```python
from build123d import *

# Parameters (mm, degrees)
SKETCH3_W                       = 111.348371095
SKETCH3_H                       = 23.1
BOSS_EXTRUDE1_DEPTH             = 5
SKETCH3_4_W                     = 34.9
SKETCH3_4_H                     = 23.1
BOSS_EXTRUDE2_DEPTH             = 2.5
CUT_EXTRUDE1_DEPTH              = 30.8
CUT_EXTRUDE1_DEPTH_BACK         = 67.894637304
SKETCH4_4_R                     = 12.7
BOSS_EXTRUDE3_START             = -1
SKETCH4_R                       = 12.7
SKETCH4_R_2                     = 4
SKETCH4_R_3                     = 1.6
BOSS_EXTRUDE3_DEPTH             = 2
BOSS_EXTRUDE4_DEPTH             = 2
BOSS_EXTRUDE4_DEPTH_BACK        = 13
BOSS_EXTRUDE4_START             = -3
SKETCH4_3_R                     = 14.8
SKETCH4_3_R_2                   = 12.7
BOSS_EXTRUDE6_REACH             = 105.413
SKETCH6_R                       = 1.7
BOSS_EXTRUDE6_DIRECTION_2_REACH = 105.413
CUT_EXTRUDE5_START              = -9.55
SKETCH6_9_R                     = 1.7
CUT_EXTRUDE5_DEPTH              = 19.1
FILLET1_R                       = 3
SKETCH12_W                      = 31.185762671
SKETCH12_H                      = 41.424107397
CUT_EXTRUDE9_DEPTH              = 2.9
FILLET2_R                       = 1
CUT_EXTRUDE10_DEPTH             = 108.072038083
FILLET3_R                       = 2
SKETCH14_W                      = 6
SKETCH14_H                      = 8
SKETCH14_R                      = 1.75
BOSS_EXTRUDE8_DEPTH             = 5
FILLET4_R                       = 10


with BuildPart() as part:
    # Sketch3 → Boss-Extrude1 (new body)
    with BuildSketch(Plane(origin=(0, 0, 0), x_dir=(1, 0, 0), z_dir=(0, 1, 0))):
        with Locations((-43.674185548, 0)):
            Rectangle(SKETCH3_W, SKETCH3_H)
    extrude(amount=-BOSS_EXTRUDE1_DEPTH)

    # Sketch3<4> → Boss-Extrude2 (add)
    with BuildSketch(Plane(origin=(0, 0, 0), x_dir=(1, 0, 0), z_dir=(0, 1, 0))):
        with Locations((-5.45, 0)):
            Rectangle(SKETCH3_4_W, SKETCH3_4_H)
        Polygon((-20.2, 9.55), (9.3, 9.55), (10, 9.55), (10, -9.55), (9.3, -9.55), (-20.2, -9.55), (-20.9, -9.55), (-20.9, 9.55), align=None, mode=Mode.SUBTRACT)
    extrude(amount=BOSS_EXTRUDE2_DEPTH)

    # Sketch4<4> → Cut-Extrude1 (cut, two sides: drawn at the far end of the back side and taken through both)
    with BuildSketch(Plane(origin=(-53.7, 0, 0), x_dir=(0, 0, -1), z_dir=(1, 0, 0)).offset(-CUT_EXTRUDE1_DEPTH_BACK)):
        with Locations((0, 9.8)):
            Circle(SKETCH4_4_R)
    extrude(amount=CUT_EXTRUDE1_DEPTH + CUT_EXTRUDE1_DEPTH_BACK, mode=Mode.SUBTRACT)

    # Sketch4 → Boss-Extrude3 (add)
    with BuildSketch(Plane(origin=(-53.7, 0, 0), x_dir=(0, 0, -1), z_dir=(1, 0, 0)).offset(BOSS_EXTRUDE3_START)):
        with Locations((0, 9.8)):
            Circle(SKETCH4_R)
        with Locations((0, 9.8)):
            Circle(SKETCH4_R_2, mode=Mode.SUBTRACT)
        with Locations((0, 18.3)):
            Circle(SKETCH4_R_3, mode=Mode.SUBTRACT)
        with Locations((0, 1.3)):
            Circle(SKETCH4_R_3, mode=Mode.SUBTRACT)
    extrude(amount=-BOSS_EXTRUDE3_DEPTH)

    # Sketch4<3> → Boss-Extrude4 (add, two sides: drawn at the far end of the back side and taken through both)
    with BuildSketch(Plane(origin=(-53.7, 0, 0), x_dir=(0, 0, -1), z_dir=(1, 0, 0)).offset(BOSS_EXTRUDE4_START - BOSS_EXTRUDE4_DEPTH_BACK)):
        with Locations((0, 9.8)):
            Circle(SKETCH4_3_R)
        with Locations((0, 9.8)):
            Circle(SKETCH4_3_R_2, mode=Mode.SUBTRACT)
    extrude(amount=BOSS_EXTRUDE4_DEPTH + BOSS_EXTRUDE4_DEPTH_BACK)

    # Boss-Extrude6: up to this face of the body (flat: up to its plane)
    boss_extrude6_end = Plane(part.part.faces().sort_by_distance((-38.495455163, -1.99193845, 11.55))[0])
    # Sketch6 → Boss-Extrude6 (add, up to the picked face)
    with BuildSketch(Plane.XY, mode=Mode.PRIVATE) as boss_extrude6_sk1:
        with BuildLine():
            Line((-22.9, 2.5), (-22.9, 3))
            ThreePointArc((-22.9, 3), (-21.435533906, 6.535533906), (-17.9, 8))
            Line((-17.9, 8), (-8.9, 8))
            Line((-8.9, 8), (0, 8))
            Line((0, 8), (0, 29))
            ThreePointArc((0, 29), (0.292893219, 29.707106781), (1, 30))
            Line((1, 30), (11, 30))
            ThreePointArc((11, 30), (11.707106781, 29.707106781), (12, 29))
            Line((12, 29), (12, 2.5))
            Line((12, 2.5), (12, 0))
            Line((12, 0), (10, 0))
            Line((10, 0), (10, 2.5))
            Line((10, 2.5), (-22.9, 2.5))
        make_face()
        with Locations(Location((-15.9, 4.5, 0), (0, 0, 180))):
            Circle(SKETCH6_R, mode=Mode.SUBTRACT)
        with Locations(Location((4.6, 25, 0), (0, 0, 180))):
            Circle(SKETCH6_R, mode=Mode.SUBTRACT)
    boss_extrude6_tool1 = split(extrude(boss_extrude6_sk1.sketch, amount=BOSS_EXTRUDE6_REACH, mode=Mode.PRIVATE), bisect_by=boss_extrude6_end, keep=Keep.BOTH, mode=Mode.PRIVATE)
    add(boss_extrude6_tool1.solids().sort_by(Axis((1.853009, 13.07203, 0), (0, 0, 1)))[0])

    # Boss-Extrude6 direction 2: up to this face of the body (flat: up to its plane)
    boss_extrude6_direction_2_end = Plane(part.part.faces().sort_by_distance((-38.495455163, -1.99193845, -11.55))[0])
    # Sketch6 → Boss-Extrude6 direction 2 (add, up to the picked face)
    with BuildSketch(Plane.XY, mode=Mode.PRIVATE) as boss_extrude6_direction_2_sk1:
        with BuildLine():
            Line((-22.9, 2.5), (-22.9, 3))
            ThreePointArc((-22.9, 3), (-21.435533906, 6.535533906), (-17.9, 8))
            Line((-17.9, 8), (-8.9, 8))
            Line((-8.9, 8), (0, 8))
            Line((0, 8), (0, 29))
            ThreePointArc((0, 29), (0.292893219, 29.707106781), (1, 30))
            Line((1, 30), (11, 30))
            ThreePointArc((11, 30), (11.707106781, 29.707106781), (12, 29))
            Line((12, 29), (12, 2.5))
            Line((12, 2.5), (12, 0))
            Line((12, 0), (10, 0))
            Line((10, 0), (10, 2.5))
            Line((10, 2.5), (-22.9, 2.5))
        make_face()
        with Locations(Location((-15.9, 4.5, 0), (0, 0, 180))):
            Circle(SKETCH6_R, mode=Mode.SUBTRACT)
        with Locations(Location((4.6, 25, 0), (0, 0, 180))):
            Circle(SKETCH6_R, mode=Mode.SUBTRACT)
    boss_extrude6_direction_2_tool1 = split(extrude(boss_extrude6_direction_2_sk1.sketch, amount=-BOSS_EXTRUDE6_DIRECTION_2_REACH, mode=Mode.PRIVATE), bisect_by=boss_extrude6_direction_2_end, keep=Keep.BOTH, mode=Mode.PRIVATE)
    add(boss_extrude6_direction_2_tool1.solids().sort_by(Axis((1.853009, 13.07203, 0), (0, 0, -1)))[0])

    # Sketch6<9> → Cut-Extrude5 (cut)
    with BuildSketch(Plane.XY.offset(CUT_EXTRUDE5_START)):
        with BuildLine():
            Line((-22.9, 2.5), (-22.9, 3))
            ThreePointArc((-22.9, 3), (-21.435533906, 6.535533906), (-17.9, 8))
            Line((-17.9, 8), (-8.9, 8))
            Line((-8.9, 8), (0, 8))
            Line((0, 8), (0, 29))
            ThreePointArc((0, 29), (0.292893219, 29.707106781), (1, 30))
            Line((1, 30), (11, 30))
            ThreePointArc((11, 30), (11.707106781, 29.707106781), (12, 29))
            Line((12, 29), (12, 2.5))
            Line((12, 2.5), (12, 0))
            Line((12, 0), (10, 0))
            Line((10, 0), (10, 2.5))
            Line((10, 2.5), (-22.9, 2.5))
        make_face()
        with Locations(Location((-15.9, 4.5, 0), (0, 0, 180))):
            Circle(SKETCH6_9_R, mode=Mode.SUBTRACT)
        with Locations(Location((4.6, 25, 0), (0, 0, 180))):
            Circle(SKETCH6_9_R, mode=Mode.SUBTRACT)
    extrude(amount=CUT_EXTRUDE5_DEPTH, mode=Mode.SUBTRACT)

    # Fillet1
    fillet1_edges = [part.edges().sort_by_distance(p)[0] for p in [
        (0, 8, -10.55),
        (0, 8, 10.55),
    ]]
    fillet(fillet1_edges, radius=FILLET1_R)

    # Sketch12 → Cut-Extrude9 (cut)
    with BuildSketch(Plane(origin=(12, 0, 0), x_dir=(0, 0, -1), z_dir=(1, 0, 0))):
        with Locations((1.113943618, 12.240146633)):
            Rectangle(SKETCH12_W, SKETCH12_H)
    extrude(amount=-CUT_EXTRUDE9_DEPTH, mode=Mode.SUBTRACT)

    # Fillet2
    fillet2_edges = [part.edges().sort_by_distance(p)[0] for p in [
        (9.1, 30, 10.55),
        (9.1, 30, -10.55),
    ]]
    fillet(fillet2_edges, radius=FILLET2_R)

    # Sketch13 → Cut-Extrude10 (cut, through all)
    with BuildSketch(Plane(origin=(0, 0, -11.55), x_dir=(-1, 0, 0), z_dir=(0, 0, -1))):
        Polygon((-4.55, 30), (0, 25), (0, 30), align=None)
    extrude(amount=-CUT_EXTRUDE10_DEPTH, mode=Mode.SUBTRACT)

    # Fillet3
    fillet3_edges = [part.edges().sort_by_distance(p)[0] for p in [
        (0, 25, 10.55),
        (4.55, 30, 10.55),
        (4.55, 30, -10.55),
        (0, 25, -10.55),
    ]]
    fillet(fillet3_edges, radius=FILLET3_R)

    # Sketch14 → Boss-Extrude8 (add)
    # profile 1 of 4: a face of its own
    with BuildSketch(Plane.XZ.offset(5)):
        with Locations((-76.348371095, -15.55)):
            Rectangle(SKETCH14_W, SKETCH14_H)
        with Locations(Location((-76.348371095, -16.55, 0), (0, 0, 270))):
            Circle(SKETCH14_R, mode=Mode.SUBTRACT)
    # profile 2 of 4: a face of its own
    with BuildSketch(Plane.XZ.offset(5)):
        with Locations((-76.348371095, 15.55)):
            Rectangle(SKETCH14_W, SKETCH14_H)
        with Locations(Location((-76.348371095, 16.55, 0), (0, 0, 270))):
            Circle(SKETCH14_R, mode=Mode.SUBTRACT)
    # profile 3 of 4: a face of its own
    with BuildSketch(Plane.XZ.offset(5)):
        with Locations((-36.348371095, -15.55)):
            Rectangle(SKETCH14_W, SKETCH14_H)
        with Locations(Location((-36.348371095, -16.55, 0), (0, 0, 270))):
            Circle(SKETCH14_R, mode=Mode.SUBTRACT)
    # profile 4 of 4: a face of its own
    with BuildSketch(Plane.XZ.offset(5)):
        with Locations((-36.348371095, 15.55)):
            Rectangle(SKETCH14_W, SKETCH14_H)
        with Locations(Location((-36.348371095, 16.55, 0), (0, 0, 270))):
            Circle(SKETCH14_R, mode=Mode.SUBTRACT)
    extrude(amount=-BOSS_EXTRUDE8_DEPTH)

    # Fillet4
    # the kernel refuses this fillet: 10 mm, written as the material it adds along each edge
    with BuildSketch(Plane(origin=(-79.348371095, -5, 11.55), x_dir=(-1, 0, 0), z_dir=(0, 1, 0)), Plane(origin=(-73.348371095, -5, -11.55), x_dir=(1, 0, 0), z_dir=(0, 1, 0)), Plane(origin=(-39.348371095, -5, 11.55), x_dir=(-1, 0, 0), z_dir=(0, 1, 0)), Plane(origin=(-33.348371095, -5, -11.55), x_dir=(1, 0, 0), z_dir=(0, 1, 0))) as fillet4_piece_1:
        with BuildLine():
            CenterArc((9.797958971, 10), FILLET4_R, 191.536959033, 78.463040967)
            Line((0, 8), (-0.195959179, 7.96))
            ThreePointArc((-0.195959179, 7.96), (-0.2, 4), (-0.2, 0))
            Line((-0.2, 0), (0, -0.2))
            Line((0, -0.2), (9.797958971, -0.2))
            Line((9.797958971, -0.2), (9.797958971, 0))
        make_face()
    extrude(amount=5)
    with BuildSketch(Plane(origin=(-73.348371095, -5, 11.55), x_dir=(1, 0, 0), z_dir=(0, 1, 0)), Plane(origin=(-79.348371095, -5, -11.55), x_dir=(-1, 0, 0), z_dir=(0, 1, 0)), Plane(origin=(-33.348371095, -5, 11.55), x_dir=(1, 0, 0), z_dir=(0, 1, 0)), Plane(origin=(-39.348371095, -5, -11.55), x_dir=(-1, 0, 0), z_dir=(0, 1, 0))) as fillet4_piece_2:
        with BuildLine():
            CenterArc((9.797958971, -10), FILLET4_R, 90, 78.463040967)
            Line((0, -8), (-0.195959179, -7.96))
            ThreePointArc((-0.195959179, -7.96), (-0.2, -4), (-0.2, 0))
            Line((-0.2, 0), (0, 0.2))
            Line((0, 0.2), (9.797958971, 0.2))
            Line((9.797958971, 0.2), (9.797958971, 0))
        make_face()
    extrude(amount=5)


solid = part.part
```
CAD build for the part. Positions are in the model's coordinates, mm. A direction names the side the tool comes from. Round coordinates to 2 decimals unless told otherwise and drop trailing zeros. Order: outer loops, then holes, each group sorted by start corner. A loop starts at its lowest first (then second) coordinate and runs counter-clockwise, first axis right, second up. Notation, with made-up numbers: (34, -8) - (85, -8) arc R26 cw to (85, 16) - close; hole circle Ø10 at (63.5, -1.75). An arc over 180 degrees is marked (long way). Use CSV: the item, a comma, the result in double quotes. Start each with the question number.
1) Two-plate mould, pull along Y, no slides. Class faces 6 (the cylindrical face through (-29.949, -2.535, -13.865)), 7 (the cylindrical face through (-68.845, -1.467, -5.86)), 8 (the flat face through (7, 30, 11)): pulls with the +Y half, pulls with the -Y half, needs draft (parallel to the pull), parting line crosses it, or undercut.
2) Pin check, flat tips, straight feed: pin 1 Ø2 at (y, z) = (17, -11) entering from -X; pin 2 Ø4.5 at (x, y) = (4.6, 25) entering from -Z; pin 3 Ø5.5 at (x, y) = (-92, -3.5) entering from +Z; pin 4 Ø3 at (x, y) = (-15.9, 4.5) entering from -Z. Stop position of each tip, or through.
3) Saw through at B-B (x = -15.9). List the corners of the cut face in (y, z).
4) Wall check: L1, parallel to X at y = -1.3, z = 16.55; L2, parallel to X at y = 13, z = -10.5; L3, parallel to X at y = 12.5, z = -4. Give the ranges that are in metal, low to high. Write a range as [from, to].
5) Tool access for faces 1 (the flat face through (-6, 0, 0)), 2 (the flat face through (-94, -2, 11.55)), 3 (the cylindrical face through (-42.748, -2.535, 13.865)), 4 (the flat face through (2.262, 27.486, 10.536)), 5 (the flat face through (0, 18, -11)): list every direction of +Z, -Z, +X, -X, +Y, -Y with a clear straight run to the whole face (end or side of a thin tool).
6) Saw through at A-A (z = 0). List the corners of the cut face in (x, y), and give its area (3 significant figures).
7) Saw through at D-D (y = 4.5). List the corners of the cut face in (x, z).
8) Saw through at C-C (y = 15.5). List the corners of the cut face in (x, z), and give its area (3 significant figures).
Values follow:
1,face 6,"needs draft"
1,face 7,"undercut"
1,face 8,"pulls with the +Y half"
2,pin 1,"stops at x = -69.7"
2,pin 2,"stops at z = -11.55"
2,pin 3,"stops at z = 11.55"
2,pin 4,"passes through"
3,outline,"(-5, -11.55) - (2.8, -11.55) - (2.8, -9.55) - (0, -9.55) - (0, 9.55) - (2.8, 9.55) - (2.8, 11.55) - (-5, 11.55) - close; (6.2, -11.55) - (8, -11.55) - (8, -9.55) - (6.2, -9.55) - close; (6.2, 9.55) - (8, 9.55) - (8, 11.55) - (6.2, 11.55) - close"
4,L1,"x = [-80.49, -78.1], [-74.6, -72.21], [-40.49, -38.1], [-34.6, -32.21]"
4,L2,"x = [-56.7, -54.7], [0, 9.1]"
4,L3,"x = [-56.7, -54.7]"
5,face 1,"+X, +Y"
5,face 2,"+Z, -X, +Y, -Y"
5,face 3,"+Z, +Y, -Y"
5,face 4,"+Z, -Z, -X, +Y"
5,face 5,"+Z, -Z, +Y"
6,outline,"(-99.35, -5) - (9.1, -5) - (9.1, 0) - (-20.9, 0) - (-20.9, 2.5) - (-22.9, 2.5) - (-22.9, -2.9) - (-54.7, -2.9) - (-54.7, -0.3) - (-56.7, -0.3) - (-56.7, -2.9) - (-99.35, -2.9) - close; (-69.7, 22.5) - (-56.7, 22.5) - (-56.7, 19.9) - (-54.7, 19.9) - (-54.7, 24.6) - (-69.7, 24.6) - close; (-56.7, 2.9) - (-54.7, 2.9) - (-54.7, 5.8) - (-56.7, 5.8) - close; (-56.7, 13.8) - (-54.7, 13.8) - (-54.7, 16.7) - (-56.7, 16.7) - close"
6,area,"379 mm2"
7,outline,"(-69.7, -13.82) - (-54.7, -13.82) - (-54.7, 13.82) - (-69.7, 13.82) - (-69.7, 11.54) - (-56.7, 11.54) - (-56.7, -11.54) - (-69.7, -11.54) - close; (-22.67, -11.55) - (-17.6, -11.55) - (-17.6, -9.55) - (-22.67, -9.55) - close; (-22.67, 9.55) - (-17.6, 9.55) - (-17.6, 11.55) - (-22.67, 11.55) - close; (-14.2, -11.55) - (9.1, -11.55) - (9.1, -9.55) - (-14.2, -9.55) - close; (-14.2, 9.55) - (9.1, 9.55) - (9.1, 11.55) - (-14.2, 11.55) - close"
8,outline,"(-69.7, -13.66) - (-54.7, -13.66) - (-54.7, 13.66) - (-69.7, 13.66) - (-69.7, 11.35) - (-56.7, 11.35) - (-56.7, -11.35) - (-69.7, -11.35) - close; (0, -11.55) - (9.1, -11.55) - (9.1, -9.55) - (0, -9.55) - close; (0, 9.55) - (9.1, 9.55) - (9.1, 11.55) - (0, 11.55) - close"
8,area,"151 mm2"
